Input: dimensioned drawing with shaded views. Units: mm. Origin: part minimum x, y, z. A direction names the side the tool comes from. Round coordinates to 2 decimals unless told otherwise and drop trailing zeros. Loops run counter-clockwise (first coordinate to the right, second up) from the corner with the lowest first, then second, coordinate; pieces in that order, holes last. Notation, with made-up numbers: (37, 89.25) - (44, 89.25) arc R15 ccw to (44, 111.25) - close; hole circle Ø5 at (-5.75, 3). An arc over 180 degrees is marked (long way). One line per question, with ' | ' between items. Start each with the question number.
Item 1: Draft query along Z for the marked faces 5, 6 and 7. Return one class per face: pulls with the +Z half, pulls with the -Z half, needs draft (parallel to the pull), parting line crosses it, or undercut.
Item 2: Material intervals for line 1 along Z through (x, y) = (1.05, 4.9); line 2 along X through (y, z) = (3.4, 3); line 3 along Y through (x, z) = (1.15, 4), sorted ascending.
Item 3: Section C-C, the plane z = 5.75. Return loops of the section in (x, y).
Item 4: First-contact query: pin 1 (0.8 mm diameter, centred on x = 0.5, y = 5.5, fed in from +Z); pin 2 (1.5 mm diameter, centred on y = 5, z = 4.5, fed in from +X); pin 3 (0.6 mm diameter, centred on x = 3, y = 4, fed in from -Z); pin 4 (2 mm diameter, centred on x = 5.5, y = 1, fed in from +Z). Flat tips, straight axial feed; report the tip coordinate or a pass-through.
Item 5: Section D-D, the plane y = 1.6. Return loops of the section in (x, z).
Item 6: Section A-A, the plane x = 1.9. Return loops of the section in (y, z), plus the area to 3 significant figures.
Item 7: Section B-B, the plane y = 3.1. Return loops of the section in (x, z).
Item 8: Set-up query: the marked faces 1, 2, 3 and 4. Return all of +Z, -Z, +X, -X, +Y, -Y with unobstructed straight access to the full face (end or side cutting, diameter ignored); none if empty.
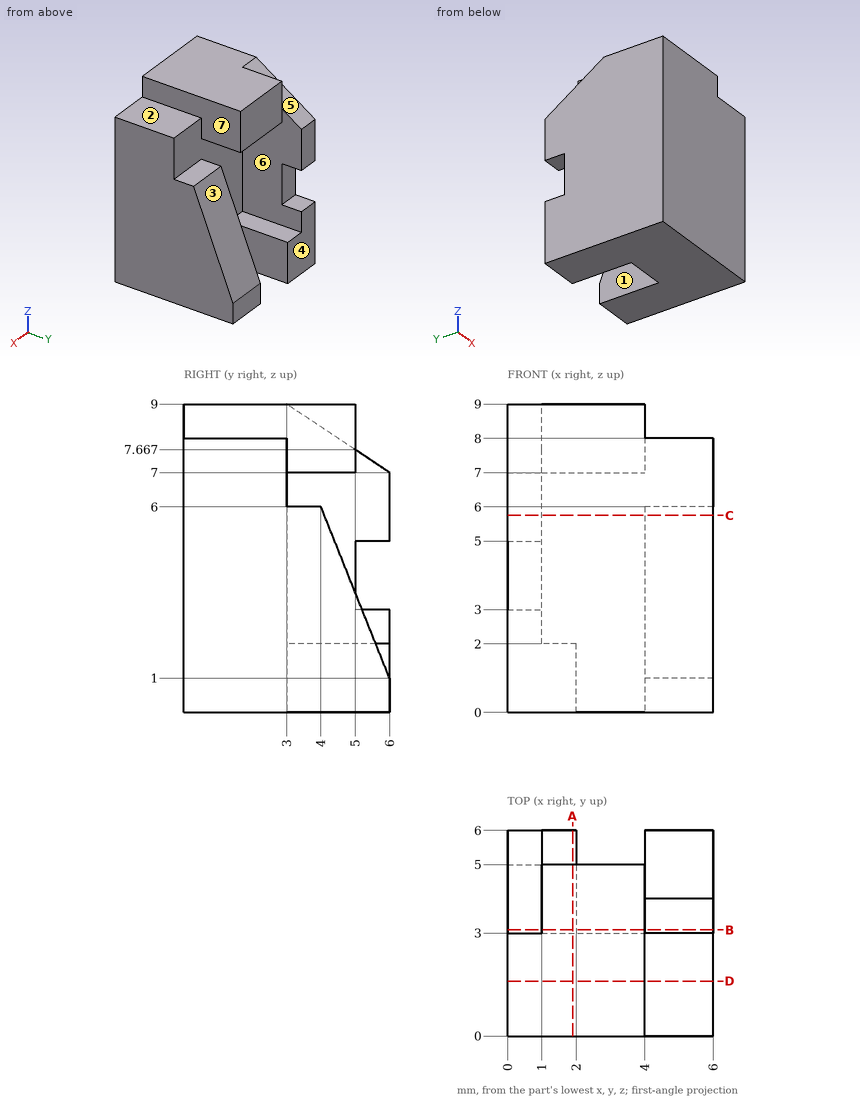
Return value:
1) face 5: pulls with the +Z half | face 6: undercut | face 7: needs draft
2) line 1: 0 to 2, 7 to 9 | line 2: 0 to 1, 4 to 6 | line 3: 0 to 3
3) outline: (0, 0) - (6, 0) - (6, 4.1) - (4, 4.1) - (4, 3) - (1, 3) - (1, 6) - (0, 6) - close
4) pin 1: z = 7.6 | pin 2: x = 6 | pin 3: z = 7 | pin 4: z = 8
5) outline: (0, 0) - (6, 0) - (6, 8) - (4, 8) - (4, 9) - (0, 9) - close
6) outline: (0, 0) - (6, 0) - (6, 2) - (3, 2) - (3, 7) - (5, 7) - (5, 9) - (0, 9) - close | area: 37.0 mm2
7) outline: (0, 0) - (2, 0) - (2, 2) - (1, 2) - (1, 7) - (4, 7) - (4, 9) - (1, 9) - (1, 8.93) - (0, 8.93) - close; (4, 0) - (6, 0) - (6, 6) - (4, 6) - close
8) face 1: -Z, +Y | face 2: +Z, +X, +Y, -Y | face 3: +Z, +X, +Y | face 4: +Z, -Z, +X, -X, +Y
